from build123d import *

# Parameters (mm, degrees)
BOSS_EXTRUDE1_DEPTH = 1.524


with BuildPart() as part:
    # Model → Boss-Extrude1 (new body)
    with BuildSketch(Plane.XY):
        with BuildLine():
            Line((134.96008858, 18.319511963), (129.201538518, 16.231235276))
            ThreePointArc((129.201538518, 16.231235276), (125.494314224, 14.202109959), (122.342593367, 11.386525267))
            ThreePointArc((122.342593367, 11.386525267), (122.521547644, 13.015286897), (121.637755911, 14.395069943))
            ThreePointArc((121.637755911, 14.395069943), (120.558535261, 14.894839146), (119.655012959, 15.668230327))
            ThreePointArc((119.655012959, 15.668230327), (116.945656671, 16.627230011), (114.111435919, 16.150276533))
            ThreePointArc((114.111435919, 16.150276533), (110.130348083, 14.492411945), (106.116427247, 12.915701804))
            ThreePointArc((106.116427247, 12.915701804), (100.871077069, 8.483544727), (94.612309809, 5.65767367))
            ThreePointArc((94.612309809, 5.65767367), (96.234412345, 7.167311858), (96.088279041, 9.378390589))
            ThreePointArc((96.088279041, 9.378390589), (87.959563224, 6.916430033), (79.738932416, 4.781365698))
            ThreePointArc((79.738932416, 4.781365698), (70.087015382, 0.573629162), (59.825334355, -1.784855875))
            ThreePointArc((59.825334355, -1.784855875), (61.625546567, -0.674388225), (62.177186804, 1.367570505))
            ThreePointArc((62.177186804, 1.367570505), (56.69945513, 0.613180121), (51.20394484, 0.001611808))
            ThreePointArc((51.20394484, 0.001611808), (42.783253785, -1.45847583), (34.430253575, 0.349086412))
            ThreePointArc((34.430253575, 0.349086412), (35.242407465, 0.582998344), (35.696308866, 1.295937508))
            ThreePointArc((35.696308866, 1.295937508), (26.899874012, 2.912690878), (18.24226034, 5.156991018))
            ThreePointArc((18.24226034, 5.156991018), (8.327270493, 6.613476825), (-1.186477097, 9.762600728))
            ThreePointArc((-1.186477097, 9.762600728), (0.567723509, 9.933888345), (2.129376981, 10.751077214))
            ThreePointArc((2.129376981, 10.751077214), (-4.564424076, 14.67509235), (-8.866303828, 21.132545253))
            ThreePointArc((-8.866303828, 21.132545253), (-2.028267146, 21.342243043), (4.458921798, 23.51459164))
            ThreePointArc((4.458921798, 23.51459164), (5.978589155, 24.100559155), (7.508094135, 24.660346004))
            ThreePointArc((7.508094135, 24.660346004), (6.073839254, 25.435989759), (4.458921798, 25.661271599))
            ThreePointArc((4.458921798, 25.661271599), (11.846812063, 27.976344953), (19.588212991, 28.082169784))
            ThreePointArc((19.588212991, 28.082169784), (24.23969735, 28.951914388), (28.92877134, 29.588583491))
            ThreePointArc((28.92877134, 29.588583491), (30.250891965, 29.696247396), (31.57341018, 29.798912074))
            ThreePointArc((31.57341018, 29.798912074), (29.710039, 31.839896858), (27.095456614, 32.73529062))
            ThreePointArc((27.095456614, 32.73529062), (46.017315853, 33.521760077), (64.749650783, 30.73699449))
            ThreePointArc((64.749650783, 30.73699449), (71.265909378, 30.552300799), (77.77761193, 30.246575893))
            ThreePointArc((77.77761193, 30.246575893), (78.240878226, 31.474299031), (77.877808016, 32.73529062))
            ThreePointArc((77.877808016, 32.73529062), (91.368554355, 30.154894712), (105.083859187, 29.413886469))
            ThreePointArc((105.083859187, 29.413886469), (112.860951548, 29.721873992), (120.624125013, 30.279690879))
            ThreePointArc((120.624125013, 30.279690879), (120.101426826, 31.522338532), (119.655012959, 32.794384617))
            ThreePointArc((119.655012959, 32.794384617), (125.469075261, 29.850060932), (131.706292975, 27.960754811))
            ThreePointArc((131.706292975, 27.960754811), (135.079830026, 28.186864843), (137.333813614, 25.666659301))
            ThreePointArc((137.333813614, 25.666659301), (137.306373673, 25.392750403), (137.099398505, 25.211255734))
            Line((137.099398505, 25.211255734), (128.692975928, 22.19615093))
            Line((128.692975928, 22.19615093), (129.201538518, 20.777960276))
            Line((129.201538518, 20.777960276), (137.683967254, 23.82080051))
            ThreePointArc((137.683967254, 23.82080051), (138.003306934, 23.78963562), (138.181844931, 23.523039923))
            ThreePointArc((138.181844931, 23.523039923), (137.524769068, 20.330730705), (134.96008858, 18.319511963))
        make_face()
        with BuildLine():
            ThreePointArc((113.344379689, 22.19615093), (96.963122218, 12.553503985), (77.990394499, 11.386525267))
            ThreePointArc((77.990394499, 11.386525267), (96.271224533, 14.816426058), (113.344379689, 22.19615093))
        make_face(mode=Mode.SUBTRACT)
        with BuildLine():
            ThreePointArc((113.344379689, 23.82080051), (96.187450512, 17.719248724), (77.990394499, 17.043744891))
            ThreePointArc((77.990394499, 17.043744891), (95.848162694, 19.489217449), (113.344379689, 23.82080051))
        make_face(mode=Mode.SUBTRACT)
        with BuildLine():
            ThreePointArc((112.010038699, 26.273742515), (95.04541072, 22.055495603), (77.613248587, 23.363904105))
            ThreePointArc((77.613248587, 23.363904105), (94.856261251, 24.29140484), (112.010038699, 26.273742515))
        make_face(mode=Mode.SUBTRACT)
        with BuildLine():
            ThreePointArc((73.920433764, 9.144198092), (59.762067232, 3.425519676), (44.552717894, 4.781365698))
            ThreePointArc((44.552717894, 4.781365698), (44.052345371, 5.659967485), (44.86760609, 6.258017419))
            ThreePointArc((44.86760609, 6.258017419), (59.284947166, 6.637177896), (73.189879005, 10.465540071))
            ThreePointArc((73.189879005, 10.465540071), (74.143785851, 10.130315533), (73.920433764, 9.144198092))
        make_face(mode=Mode.SUBTRACT)
        with BuildLine():
            ThreePointArc((73.7171882, 14.19085222), (74.195068041, 15.63804442), (72.809895852, 16.27367986))
            ThreePointArc((72.809895852, 16.27367986), (57.603683966, 13.161162203), (42.082533848, 13.058472776))
            ThreePointArc((42.082533848, 13.058472776), (41.678568271, 12.772614258), (41.897709615, 12.328902245))
            ThreePointArc((41.897709615, 12.328902245), (58.027223609, 9.504074716), (73.7171882, 14.19085222))
        make_face(mode=Mode.SUBTRACT)
        with BuildLine():
            ThreePointArc((71.615953494, 19.263251529), (72.005249, 20.227653753), (71.069824737, 20.682190977))
            ThreePointArc((71.069824737, 20.682190977), (55.942470801, 18.367444511), (40.793050931, 20.533077418))
            ThreePointArc((40.793050931, 20.533077418), (39.862149142, 20.069348511), (40.260924923, 19.10882755))
            ThreePointArc((40.260924923, 19.10882755), (55.955346454, 15.753106638), (71.615953494, 19.263251529))
        make_face(mode=Mode.SUBTRACT)
        with BuildLine():
            ThreePointArc((75.249897816, 23.419828185), (57.358073705, 25.777828917), (39.34157015, 24.737090166))
            ThreePointArc((39.34157015, 24.737090166), (57.468271047, 28.781788902), (75.249897816, 23.419828185))
        make_face(mode=Mode.SUBTRACT)
        with BuildLine():
            ThreePointArc((38.218093055, 8.509361046), (23.165664514, 8.263848957), (8.79939997, 12.763440518))
            ThreePointArc((8.79939997, 12.763440518), (22.937130999, 6.683446576), (38.218093055, 8.509361046))
        make_face(mode=Mode.SUBTRACT)
        with BuildLine():
            ThreePointArc((37.366333435, 14.19085222), (23.1546149, 13.598745989), (9.184351398, 16.27367986))
            ThreePointArc((9.184351398, 16.27367986), (22.976923316, 11.194465897), (37.366333435, 14.19085222))
        make_face(mode=Mode.SUBTRACT)
        with BuildLine():
            ThreePointArc((36.84813704, 17.413649418), (23.030567399, 17.299167045), (9.596276919, 20.533077418))
            ThreePointArc((9.596276919, 20.533077418), (23.40846607, 20.600554903), (36.84813704, 17.413649418))
        make_face(mode=Mode.SUBTRACT)
        with BuildLine():
            ThreePointArc((35.94161169, 23.51459164), (22.768944305, 24.649665002), (9.596276919, 23.51459164))
            ThreePointArc((9.596276919, 23.51459164), (22.768944305, 27.614666916), (35.94161169, 23.51459164))
        make_face(mode=Mode.SUBTRACT)
    extrude(amount=BOSS_EXTRUDE1_DEPTH)


solid = part.part
Verification items for the finished model (mm, model axes). A direction names the side the tool comes from. Round coordinates to 2 decimals unless told otherwise and drop trailing zeros. Loops run counter-clockwise (first coordinate to the right, second up) from the corner with the lowest first, then second, coordinate; pieces in that order, holes last. Notation, with made-up numbers: (28, 40.25) - (59, 40.25) arc R20 ccw to (59, 70.25) - close; hole circle Ø6 at (84.5, 82). An arc over 180 degrees is marked (long way). Use a Markdown table: item, result. Add a question column.
1. Release check for a two-part mould opening along X. For faces 1 (the face through (66, 16, 0)), 2 (the face through (95.29, 22.077, 0.751)), 3 (the face through (45.752, 33.535, 0.751)), 4 (the face through (70.23, 0.62, 0.75)) record: released by +X, released by -X, zero draft, split by the parting line, or undercut.
2. Gauge pin test, flat end, axial feed: pin 1 (12 mm diameter, centred on x = 84, y = 12, fed in from -Z). Record the tip position at first contact, or that the pin passes through.
3. Thickness scan on probe 1 along Y at (x, z) = (63, 0.7); probe 2 along Y at (x, z) = (43, 1.25); probe 3 along Y at (x, z) = (44, 0.7). Record the ranges inside material, lowest first. Write a range as [from, to].
4. Section check A-A, the plane x = 68. Record the boundary of the cut face in (y, z), plus the area to 3 significant figures.
5. Section check D-D, the plane x = 17. Record the boundary of the cut face in (y, z), plus the area to 3 significant figures.
6. Access from +Z, -Z, +X, -X, +Y, -Y to the whole of each face (thin tool, end or side, straight path). Record for faces 5 (the face through (132.955, 23.725, 0.751)), 6 (the face through (110.186, 14.515, 0.751)), 7 (the face through (135.034, 28.205, 0.751)).
7. Section check C-C, the plane z = 0.55. Give the number of separate pieces and of enclosed holes in the cut face, plus the area to 3 significant figures.
8. Section check B-B, the plane x = 84. Record the boundary of the cut face in (y, z), plus the area to 3 significant figures.
Checks:
| question | item | result |
|---|---|---|
| 1 | face 1 | zero draft |
| 1 | face 2 | undercut |
| 1 | face 3 | undercut |
| 1 | face 4 | released by +X |
| 2 | pin 1 | stops at z = 0 |
| 3 | probe 1 | y = [-1.27, 4.08], [7.31, 10.15], [13.91, 16.46], [18.88, 25.4], [28.16, 31.15] |
| 3 | probe 2 | y = [-1.46, 11.88], [12.98, 17.99], [19.93, 25.23], [26.38, 33.64] |
| 3 | probe 3 | y = [-1.45, 11.5], [12.91, 17.65], [19.69, 25.33], [26.74, 33.61] |
| 4 | outline | (-0.07, 0) - (5.79, 0) - (5.79, 1.52) - (-0.07, 1.52) - close; (8.61, 0) - (11.54, 0) - (11.54, 1.52) - (8.61, 1.52) - close; (14.95, 0) - (17.8, 0) - (17.8, 1.52) - (14.95, 1.52) - close; (19.84, 0) - (24.79, 0) - (24.79, 1.52) - (19.84, 1.52) - close; (26.83, 0) - (30.66, 0) - (30.66, 1.52) - (26.83, 1.52) - close |
| 4 | area | 31.1 mm^2 |
| 5 | outline | (5.24, 0) - (8.18, 0) - (8.18, 1.52) - (5.24, 1.52) - close; (9.58, 0) - (12.33, 0) - (12.33, 1.52) - (9.58, 1.52) - close; (14.37, 0) - (18.32, 0) - (18.32, 1.52) - (14.37, 1.52) - close; (20.98, 0) - (24.43, 0) - (24.43, 1.52) - (20.98, 1.52) - close; (26.89, 0) - (28.3, 0) - (28.3, 1.52) - (26.89, 1.52) - close |
| 5 | area | 22.1 mm^2 |
| 6 | face 5 | +Z, -Z |
| 6 | face 6 | +Z, -Z, -Y |
| 6 | face 7 | +Z, -Z, +Y |
| 7 | separate pieces | 1 |
| 7 | enclosed holes | 11 |
| 7 | area | 2,630 mm^2 |
| 8 | outline | (5.84, 0) - (10.79, 0) - (10.79, 1.52) - (5.84, 1.52) - close; (12.05, 0) - (16.65, 0) - (16.65, 1.52) - (12.05, 1.52) - close; (17.65, 0) - (22.23, 0) - (22.23, 1.52) - (17.65, 1.52) - close; (23.58, 0) - (31.33, 0) - (31.33, 1.52) - (23.58, 1.52) - close |
| 8 | area | 33.3 mm^2 |
